from build123d import *

# Parameters (mm, degrees)
BOSS_EXTRUDE2_DEPTH     = 3
CUT_EXTRUDE1_DEPTH      = 301.665110986
CUT_EXTRUDE2_DEPTH      = 301.665110986
CUT_EXTRUDE2_DEPTH_BACK = 301.665110986
SKETCH5_R               = 3.325


with BuildPart() as part:
    # Sketch3 → Boss-Extrude2 (new body)
    with BuildSketch(Plane(origin=(0, 0, 0), x_dir=(1, 0, 0), z_dir=(0, 1, 0))):
        with BuildLine():
            Line((-71.592001125, 291.800526166), (-30.005764519, 291.800526166))
            Line((-30.005764519, 291.800526166), (-30.005764519, 264.934819646))
            ThreePointArc((-30.005764519, 264.934819646), (0, 234.929055126), (30.005764519, 264.934819646))
            Line((30.005764519, 264.934819646), (30.005764519, 291.800526166))
            Line((30.005764519, 291.800526166), (72.408299895, 291.800526166))
            Line((72.408299895, 291.800526166), (72.408299895, -219.373421964))
            Line((72.408299895, -219.373421964), (0.408149385, -291.373572474))
            Line((0.408149385, -291.373572474), (-71.592001125, -219.373421964))
            Line((-71.592001125, -219.373421964), (-71.592001125, 291.800526166))
        make_face()
    extrude(amount=BOSS_EXTRUDE2_DEPTH)

    # Sketch4 → Cut-Extrude1 (cut, through all)
    with BuildSketch(Plane(origin=(0, 3, 0), x_dir=(1, 0, 0), z_dir=(0, 1, 0))):
        Polygon((-7, -283.965423089), (-7, -255.965423089), (7, -255.965423089), (7, -284.781721859), (0.408149385, -291.373572474), align=None)
    extrude(amount=-CUT_EXTRUDE1_DEPTH, mode=Mode.SUBTRACT)

    # Sketch5 → Cut-Extrude2 (cut, two sides: drawn at the far end of the back side and taken through both)
    with BuildSketch(Plane(origin=(0, 3, 0), x_dir=(1, 0, 0), z_dir=(0, 1, 0)).offset(-CUT_EXTRUDE2_DEPTH_BACK)):
        with Locations(Location((-28.65007526, -241.415105099, 0), (0, 0, 270))):
            Circle(SKETCH5_R)
        with Locations(Location((-57.30015051, -172.372698109, 0), (0, 0, 270))):
            Circle(SKETCH5_R)
        with Locations(Location((-57.30015051, -82.372698109, 0), (0, 0, 270))):
            Circle(SKETCH5_R)
        with Locations(Location((-57.30015051, 7.627301891, 0), (0, 0, 270))):
            Circle(SKETCH5_R)
        with Locations(Location((-57.30015051, 97.627301891, 0), (0, 0, 270))):
            Circle(SKETCH5_R)
        with Locations(Location((-57.30015051, 187.627301891, 0), (0, 0, 270))):
            Circle(SKETCH5_R)
        with Locations(Location((57.30015051, 187.627301891, 0), (0, 0, 90))):
            Circle(SKETCH5_R)
        with Locations(Location((57.30015051, 97.627301891, 0), (0, 0, 90))):
            Circle(SKETCH5_R)
        with Locations(Location((57.30015051, -82.372698109, 0), (0, 0, 90))):
            Circle(SKETCH5_R)
        with Locations(Location((57.30015051, -172.372698109, 0), (0, 0, 90))):
            Circle(SKETCH5_R)
        with Locations(Location((57.30015051, 7.627301891, 0), (0, 0, 90))):
            Circle(SKETCH5_R)
        with Locations(Location((28.65007526, -241.415105099, 0), (0, 0, 90))):
            Circle(SKETCH5_R)
        with Locations(Location((41.537257894, 261.609819636, 0), (0, 0, 270))):
            Circle(SKETCH5_R)
        with Locations(Location((-41.537257894, 261.609819636, 0), (0, 0, 90))):
            Circle(SKETCH5_R)
    extrude(amount=CUT_EXTRUDE2_DEPTH + CUT_EXTRUDE2_DEPTH_BACK, mode=Mode.SUBTRACT)


solid = part.part
Verification items for the finished model (mm, model axes). Give positions to 0.01 mm unless a question says otherwise; leave off trailing zeros. Loops run counter-clockwise (first coordinate to the right, second up) from the corner with the lowest first, then second, coordinate; pieces in that order, holes last.
1. Go/stop test with flat-tipped pins: P1, Ø0.9, axis at x = -1.5, y = 2, coming from the +Z side; P2, Ø1.5, axis at y = 1, z = 263, coming from the +X side; P3, Ø1.5, axis at y = 2, z = 266, coming from the -X side. Record where each tip stops, or that it passes through.
Derived:
P1: stops at z = 255.97
P2: stops at x = 29.53
P3: stops at x = -25.72
2. Release check for a two-part mould opening along X. For faces 1 (the flat face through (1, 3, -8)), 2 (the cylindrical face through (-0.66, 1.479, -234.936)), 3 (the flat face through (40.16, 1.48, 251.62)) record: +X half, -X half, draft (parallel to the pull), parting line (faces both ways), or undercut.
Derived:
face 1: draft
face 2: undercut
face 3: +X half
3. Cross-section at A-A on x = 0. Record the cut outline in (y, z), and give its area (3 significant figures).
Derived:
outline: (0, -234.93) - (3, -234.93) - (3, 255.97) - (0, 255.97) - close
area: 1,470 mm2
4. Cross-section at B-B on y = 1. Count the separate pieces of the cut face and the enclosed holes in it, and give its area (3 significant figures).
Derived:
separate pieces: 1
enclosed holes: 14
area: 74,800 mm2
5. Material ranges on probe 1 along Z at (x, y) = (-58, 0.8); probe 2 along X at (y, z) = (0.75, 83.5); probe 3 along Z at (x, y) = (42, 2.6), recorded low to high.
Derived:
probe 1: z = -291.8 to -190.88, -184.38 to -100.88, -94.38 to -10.88, -4.38 to 79.12, 85.62 to 169.12, 175.62 to 232.97
probe 2: x = -71.59 to -60.43, -54.17 to 54.17, 60.43 to 72.41
probe 3: z = -291.8 to -264.9, -258.32 to 249.78
